from build123d import *

# Parameters (mm, degrees)
EXTRUDE_1_DEPTH = 100
SKETCH_3_W      = 100
SKETCH_3_H      = 100
EXTRUDE_3_DEPTH = 100


with BuildPart() as part:
    # 草图1 → 凸台-拉伸1 (new body)
    with BuildSketch(Plane(origin=(0, 0, 0), x_dir=(1, 0, 0), z_dir=(0, 1, 0))):
        Polygon((0, 0), (200, 0), (200, 100), (100, 100), (100, 200), (0, 200), align=None)
    extrude(amount=EXTRUDE_1_DEPTH)

    # 草图3 → 凸台-拉伸3 (add)
    with BuildSketch(Plane.ZY):
        with Locations((-50, 50)):
            Rectangle(SKETCH_3_W, SKETCH_3_H)
    extrude(amount=EXTRUDE_3_DEPTH)


solid = part.part
Can you work these out from the model? Positions are in its coordinate system, mm. A direction names the side the tool comes from. Give positions to 0.01 mm unless a question says otherwise; leave off trailing zeros. Loops run counter-clockwise (first coordinate to the right, second up) from the corner with the lowest first, then second, coordinate; pieces in that order, holes last. Notation, with made-up numbers: (56, 9.5) - (76, 9.5) arc R29 cw to (76, 48.5) - close; hole circle Ø10 at (1.5, 46.25). An arc over 180 degrees is marked (long way). One line per item, written item: value.
(1) On a 3-axis mill with a long thin cutter (end or side, diameter ignored), from which of +Z, -Z, +X, -X, +Y, -Y can I reach the whole of each face in a straight line? I mean faces 1 (the face through (52, 49, 0)), 2 (the face through (100, 49, -149)), 3 (the face through (-49, 49, -100)). Say none if no direction works.
Verdict:
face 1: +Z, +X, -X, +Y, -Y
face 2: -Z, +X, +Y, -Y
face 3: -Z, -X, +Y, -Y
(2) I'm going to push a flat-ended pin straight in: pin 1 (3 mm diameter, centred on y = 47, z = -149, fed in from -X). Where does the tip first touch, or does it pass through?
Verdict:
pin 1: x = 0
(3) If we section it at A-A, the plane y = 11.5: List the corners of the cut face in (x, z) for me.
Verdict:
outline: (-100, -100) - (0, -100) - (0, -200) - (100, -200) - (100, -100) - (200, -100) - (200, 0) - (-100, 0) - close
(4) If we section it at C-C, the plane z = -143: List the corners of the cut face in (x, y) for me, plus the area to 3 significant figures.
Verdict:
outline: (0, 0) - (100, 0) - (100, 100) - (0, 100) - close
area: 10,000 mm^2
(5) I need wall thicknesses on line 1 along X through (y, z) = (35, -109.5); line 2 along Z through (x, y) = (153.5, 48.5). Which ranges of each line are inside material? Lowest first, please.
Verdict:
line 1: 0 to 100
line 2: -100 to 0
(6) If we section it at B-B, the plane x = -26: List the corners of the cut face in (y, z) for me, plus the area to 3 significant figures.
Verdict:
outline: (0, -100) - (100, -100) - (100, 0) - (0, 0) - close
area: 10,000 mm^2
